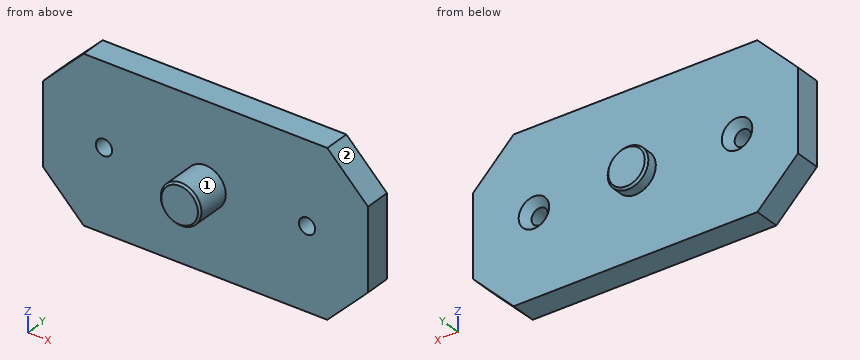
from build123d import *

# Parameters (mm, degrees)
SKETCH1_W                                       = 80
SKETCH1_H                                       = 40
BOSS_EXTRUDE1_DEPTH                             = 6.35
CSK_FOR_M3_FLAT_HEAD_MACHINE_SCREW1_D           = 4
CSK_FOR_M3_FLAT_HEAD_MACHINE_SCREW1_CSINK_D     = 7.5
CSK_FOR_M3_FLAT_HEAD_MACHINE_SCREW1_CSINK_ANGLE = 85
BOSS_EXTRUDE2_DEPTH                             = 3
BOSS_EXTRUDE2_DEPTH_BACK                        = 15
SKETCH8_R                                       = 5
CHAMFER1_SIZE                                   = 10
CHAMFER2_SIZE                                   = 0.5


with BuildPart() as part:
    # Sketch1 → Boss-Extrude1 (new body)
    with BuildSketch(Plane(origin=(0, 0, 0), x_dir=(1, 0, 0), z_dir=(0, 1, 0))):
        Rectangle(SKETCH1_W, SKETCH1_H)
    extrude(amount=BOSS_EXTRUDE1_DEPTH)

    # CSK for M3 Flat Head Machine Screw1 (through all)
    with Locations(Plane(origin=(0, 6.35, 0), x_dir=(1, 0, 0), z_dir=(0, 1, 0))):
        with Locations((-25, 0), (25, 0)):
            CounterSinkHole(CSK_FOR_M3_FLAT_HEAD_MACHINE_SCREW1_D / 2, CSK_FOR_M3_FLAT_HEAD_MACHINE_SCREW1_CSINK_D / 2, counter_sink_angle=CSK_FOR_M3_FLAT_HEAD_MACHINE_SCREW1_CSINK_ANGLE)

    # Sketch8 → Boss-Extrude2 (add, two sides: drawn at the far end of the back side and taken through both)
    with BuildSketch(Plane(origin=(0, 6.35, 0), x_dir=(1, 0, 0), z_dir=(0, 1, 0)).offset(-BOSS_EXTRUDE2_DEPTH_BACK)):
        with Locations(Location((0, 0, 0), (0, 0, 270))):
            Circle(SKETCH8_R)
    extrude(amount=BOSS_EXTRUDE2_DEPTH + BOSS_EXTRUDE2_DEPTH_BACK)

    # Chamfer1
    chamfer1_edges = [part.edges().sort_by_distance(p)[0] for p in [
        (40, 3.175, 20),
        (-40, 3.175, 20),
        (-40, 3.175, -20),
        (40, 3.175, -20),
    ]]
    chamfer(chamfer1_edges, length=CHAMFER1_SIZE)

    # Chamfer2
    chamfer2_edges = [part.edges().sort_by_distance(p)[0] for p in [
        (0, -8.65, -5),
        (0, 9.35, -5),
    ]]
    chamfer(chamfer2_edges, length=CHAMFER2_SIZE)


solid = part.part
Can you work these out from the model? Positions are in its coordinate system, mm. Face numbers are marked on the shaded views. A direction names the side the tool comes from. Give positions to 0.01 mm unless a question says otherwise; leave off trailing zeros. Order: outer loops, then holes, each group sorted by start corner. A loop starts at its lowest first (then second) coordinate and runs counter-clockwise, first axis right, second up. Notation, with made-up numbers: M -9.75,-33 L -4.75,-33 A29 ccw -4.75,-5 Z; hole C 51.25,87 d1. An arc over 180 degrees is marked long. Use a Markdown table: item, result. Add a question column.
Item 1: Suppose I cut it at D-D (x = 0). List the corners of the cut face in (y, z) for me.
Item 2: Will these pins go through, and if not, where does the flat tip stop? pin 1 (1 mm diameter, centred on y = -6.5, z = -0.5, fed in from +X); pin 2 (2 mm diameter, centred on x = 27, z = -10.5, fed in from +Y).
Item 3: If I drill on L1, parallel to Z at x = -25, y = 1.7; L2, parallel to Y at x = 16, z = -14; L3, parallel to Z at x = 4.5, y = -4.75, over which ranges is the centre line in solid material (lowest first)? Write a range as [from, to].
Item 4: For the marked faces 1 and 2, which set-ups out of +Z, -Z, +X, -X, +Y, -Y let a thin tool reach every point of the face, with its end or its side?
Item 5: Suppose I cut it at A-A (z = 0). List the corners of the cut face in (x, y) for me.
Item 6: Suppose I cut it at C-C (y = 1.5). List the corners of the cut face in (x, z) for me.
Item 7: Suppose I cut it at B-B (x = -25). List the corners of the cut face in (y, z) for me.
Answer sheet:
| question | item | result |
|---|---|---|
| 1 | outline | M -8.65,-4.5 L -8.15,-5 L 0,-5 L 0,-20 L 6.35,-20 L 6.35,-5 L 8.85,-5 L 9.35,-4.5 L 9.35,4.5 L 8.85,5 L 6.35,5 L 6.35,20 L 0,20 L 0,5 L -8.15,5 L -8.65,4.5 Z |
| 2 | pin 1 | stops at x = 5 |
| 2 | pin 2 | stops at y = 6.35 |
| 3 | L1 | z = [-20, -2], [2, 20] |
| 3 | L2 | y = [0, 6.35] |
| 3 | L3 | z = [-2.18, 2.18] |
| 4 | face 1 | -Y |
| 4 | face 2 | +Z, +X, +Y, -Y |
| 5 | outline | M -40,0 L -27,0 L -27,4.44 L -28.75,6.35 L -40,6.35 Z; M -23,0 L -5,0 L -5,-8.15 L -4.5,-8.65 L 4.5,-8.65 L 5,-8.15 L 5,0 L 23,0 L 23,4.44 L 21.25,6.35 L 5,6.35 L 5,8.85 L 4.5,9.35 L -4.5,9.35 L -5,8.85 L -5,6.35 L -21.25,6.35 L -23,4.44 Z; M 27,0 L 40,0 L 40,6.35 L 28.75,6.35 L 27,4.44 Z |
| 6 | outline | M -40,-10 L -30,-20 L 30,-20 L 40,-10 L 40,10 L 30,20 L -30,20 L -40,10 Z; hole C -25,0 d4; hole C 25,0 d4 |
| 7 | outline | M 0,-20 L 6.35,-20 L 6.35,-3.75 L 4.44,-2 L 0,-2 Z; M 0,2 L 4.44,2 L 6.35,3.75 L 6.35,20 L 0,20 Z |
